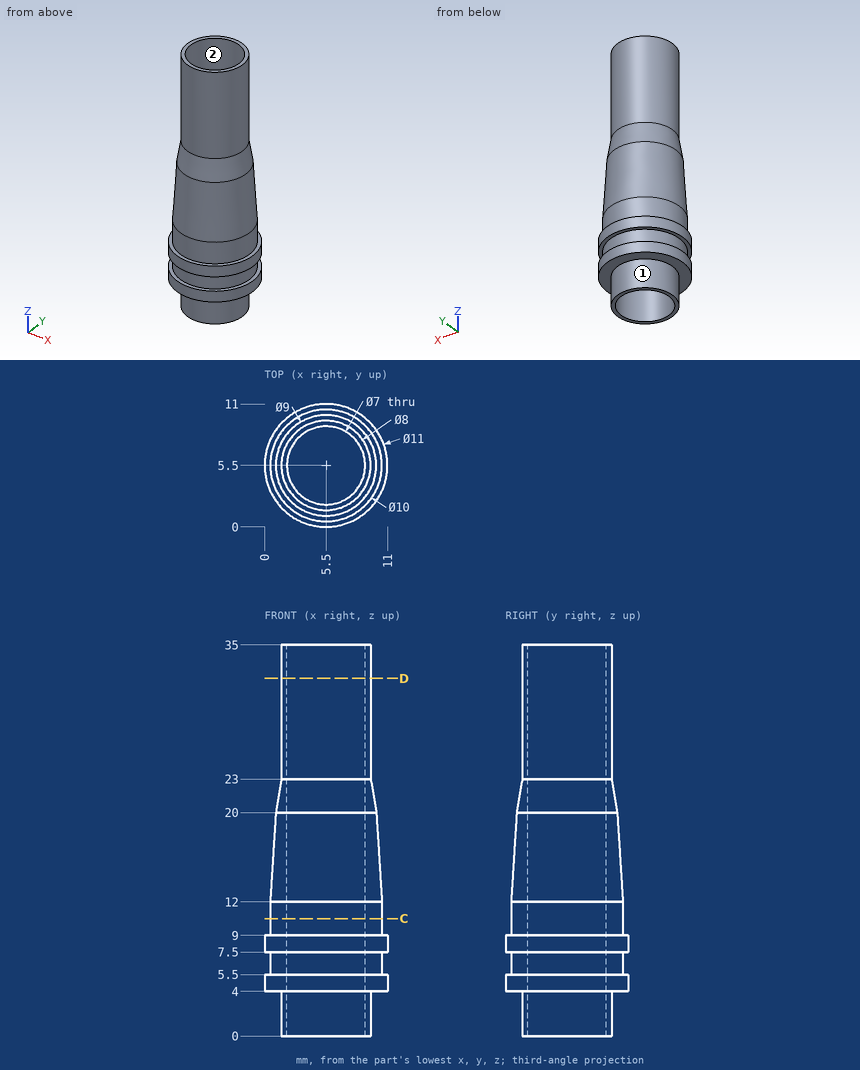
Geometry: see drawing. Coordinates: mm, zero at the bounding-box minimum. Give positions to 0.01 mm unless a question says otherwise; leave off trailing zeros. Order: outer loops, then holes, each group sorted by start corner. A loop starts at its lowest first (then second) coordinate and runs counter-clockwise, first axis right, second up. Notation, with made-up numbers: (3, 71.5) -> (28, 71.5) arc R28 ccw to (28, 104.5) -> close; hole circle Ø3 at (46, 55.5). An arc over 180 degrees is marked (long way). Write each question's results on one line, items separated by ' | '.
1) Cut plane C-C (z = 10.5). Output: boundary loops of the cut face in (x, y).
Geometry says:
outline: circle Ø10 at (5.5, 5.5); hole circle Ø7 at (5.5, 5.5)
2) Line query: line 1 along Z through (x, y) = (2.5, 10); line 2 along Y through (x, z) = (5.5, 25.5); line 3 along Y through (x, z) = (8.5, 2.5). Output: solid intervals per line, ascending.
Geometry says:
line 1: z = 4 to 5.5, 7.5 to 9 | line 2: y = 1.5 to 2, 9 to 9.5 | line 3: y = 2.85 to 3.7, 7.3 to 8.15
3) Draft query along X for the marked faces 1 and 2. Return one class per face: released by +X, released by -X, zero draft, split by the parting line, or undercut.
Geometry says:
face 1: split by the parting line | face 2: undercut
4) Cut plane D-D (z = 32). Output: boundary loops of the cut face in (x, y), and give its area (3 significant figures).
Geometry says:
outline: circle Ø8 at (5.5, 5.5); hole circle Ø7 at (5.5, 5.5) | area: 11.8 mm²
5) First-contact query: pin 1 Ø2 at (y, z) = (9.5, 27.5) entering from +X; pin 2 Ø1 at (x, y) = (7.5, 4) entering from -Z; pin 3 Ø1 at (y, z) = (8, 28) entering from +X; pin 4 Ø1.5 at (y, z) = (3.5, 22) entering from +X. Flat tips, straight axial feed; report the tip coordinate or a pass-through.
Geometry says:
pin 1: stops at x = 8.15 | pin 2: passes through | pin 3: stops at x = 8.96 | pin 4: stops at x = 9.51
